Here's how the part is built. I have some questions about the finished solid (model axes, mm). Face numbers are marked on the shaded views. A direction names the side the tool comes from. Coordinates: 2 decimals unless noted, no trailing zeros. Loops run counter-clockwise (first coordinate to the right, second up) from the corner with the lowest first, then second, coordinate; pieces in that order, holes last. Notation, with made-up numbers: (8.5, 15.5) -> (23.5, 15.5) arc R29 ccw to (23.5, 40.5) -> close; hole circle Ø6 at (1.25, 5.5). An arc over 180 degrees is marked (long way). Answer as a JSON object with one key per item and string values. Group by question number.
Q1. I'm going to push flat-ended pins straight in: pin 1 (5 mm diameter, centred on y = 19, z = 25, fed in from +X); pin 2 (1.5 mm diameter, centred on x = 39.5, z = 26.5, fed in from -Y); pin 3 (12 mm diameter, centred on x = 89, z = -15.5, fed in from +Y). Where does each tip first touch, or does it pass through?
Q2. On a 3-axis mill with a long thin cutter (end or side, diameter ignored), from which of +Z, -Z, +X, -X, +Y, -Y can I reach the whole of each face in a straight line? I mean the marked faces 1 and 2. Say none if no direction works.
Q3. I want a section at B-B on z = -26.5. Write out the boundary of the cut face in (x, y).
Q4. I want a section at D-D on z = 23. Write out the boundary of the cut face in (x, y).
Q5. I want a section at A-A on x = 83. Write out the boundary of the cut face in (y, z), then the cut area to 3 significant figures.
Q6. Thinking about a two-plate mould opening in X: for the marked faces 3, 4 and 5, which applies, released by +X, released by -X, zero draft, split by the parting line, or undercut?
Q7. I need wall thicknesses on line 1 (Z direction, x = 80, y = 2.5); line 2 (Y direction, x = 4.75, z = 30); line 3 (X direction, y = 14, z = -24). Which ranges of each line are inside material? Lowest first, please.
Q8. I want a section at C-C on x = 8.5. Write out the boundary of the cut face in (y, z).
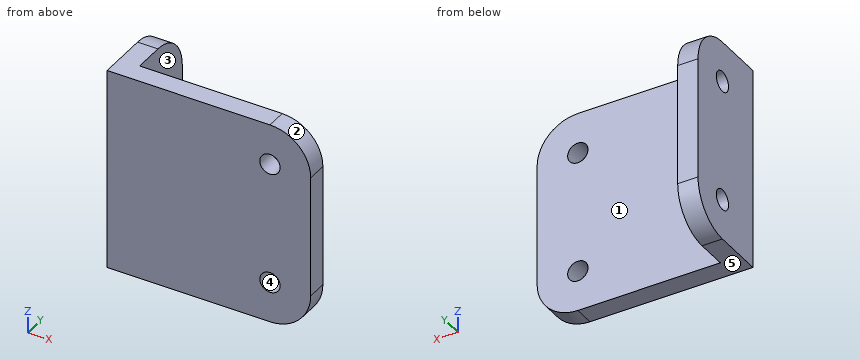
Autodesk Fusion 360 part; units mm, degrees
sketch "Sketch1" plane through (0, 0, 0) normal (0, 0, 1) x (1, 0, 0)
  line L0 (0, 0) -> (0, 45)
  line L1 (0, 45) -> (10, 45)
  line L2 (10, 45) -> (10, 10)
  line L3 (10, 10) -> (100, 10)
  line L4 (100, 10) -> (100, 0)
  line L5 (100, 0) -> (0, 0)
  dimension "d1" = 10
  dimension "d2" = 100
  dimension "d3" = 45
extrude "Extrude1" add sketch "Sketch1" along normal mid plane 100
fillet "Fillet1" radius 20 4 edges at (5, 45, 50) (5, 45, -50) (100, 5, -50) (100, 5, 50)
sketch "Sketch2" plane through (10, 0, 0) normal (1, 0, 0) x (0, 0, -1)
  arc A0 (50, 25) -> (30, 45) centre (30, 25) ccw
  line L0 (30, 45) -> (-30, 45)
  arc A1 (-30, 45) -> (-50, 25) centre (-30, 25) ccw
  line L1 (-50, 25) -> (-50, 10)
  line L2 (-50, 10) -> (50, 10)
  line L3 (50, 10) -> (50, 25)
  circle A2 centre (-30, 25) radius 10
  circle A3 centre (30, 25) radius 10
  dimension "d7" = 20
extrude "Extrude2" cut sketch "Sketch2" against normal through all contours A2 | A3
sketch "Sketch3" plane through (0, 10, 0) normal (0, 1, 0) x (-1, 0, 0)
  arc A0 (-80, 50) -> (-100, 30) centre (-80, 30) ccw
  line L0 (-100, 30) -> (-100, -30)
  arc A1 (-100, -30) -> (-80, -50) centre (-80, -30) ccw
  line L1 (-80, -50) -> (-10, -50)
  line L2 (-10, -50) -> (-10, 50)
  line L3 (-10, 50) -> (-80, 50)
  circle A2 centre (-80, -30) radius 10
  circle A3 centre (-80, 30) radius 10
  dimension "d9" = 20
extrude "Extrude3" cut sketch "Sketch3" against normal through all contours A2 | A3
move_face "OffsetFaces1" offset 5 4 faces at (6.6667, 24.0043, 20.0497) (6.6667, 24.0043, -39.9503) (70.0497, 6.6667, -30.9957) (70.0497, 6.6667, 29.0043)
Result set:
{
 "1": {"pin 1": "stops at x = 10", "pin 2": "stops at y = 0", "pin 3": "stops at y = 10"},
 "2": {"face 1": "+Z, -Z, +X, +Y", "face 2": "+Z, +X, +Y, -Y"},
 "3": {"outline": "(0, 0) -> (76.43, 0) -> (76.43, 10) -> (10, 10) -> (10, 21.43) -> (0, 21.43) -> close; (0, 28.57) -> (10, 28.57) -> (10, 45) -> (0, 45) -> close; (83.57, 0) -> (100, 0) -> (100, 10) -> (83.57, 10) -> close"},
 "4": {"outline": "(0, 0) -> (100, 0) -> (100, 10) -> (10, 10) -> (10, 45) -> (0, 45) -> close"},
 "5": {"outline": "(0, -49.77) -> (10, -49.77) -> (10, -34) -> (0, -34) -> close; (0, -26) -> (10, -26) -> (10, 26) -> (0, 26) -> close; (0, 34) -> (10, 34) -> (10, 49.77) -> (0, 49.77) -> close", "area": "835 mm²"},
 "6": {"face 3": "released by +X", "face 4": "undercut", "face 5": "zero draft"},
 "7": {"line 1": "z = -50 to -35, -25 to 25, 35 to 50", "line 2": "y = 0 to 20, 30 to 45", "line 3": "x = 0 to 10"},
 "8": {"outline": "(0, -50) -> (25, -50) arc R20 ccw to (45, -30) -> (45, 30) arc R20 ccw to (25, 50) -> (0, 50) -> close; hole circle Ø10 at (25, -30); hole circle Ø10 at (25, 30)"}
}
